Answer from the drawing. Dimensions are ordinates in mm from the lowest x, y and z of the part. Round coordinates to 2 decimals unless told otherwise and drop trailing zeros. Write each loop counter-clockwise with the first axis right and the second up, starting at its lowest first coordinate (ties: lowest second). Pieces come first, ordered by that corner, then holes. Notation, with made-up numbers: (22, 35.5) - (51, 35.5) arc R14 cw to (51, 55.5) - close; hole circle Ø1 at (56.5, 39.5). An arc over 180 degrees is marked (long way). Return JSON: item names as keys, results as strings. Group by question number.
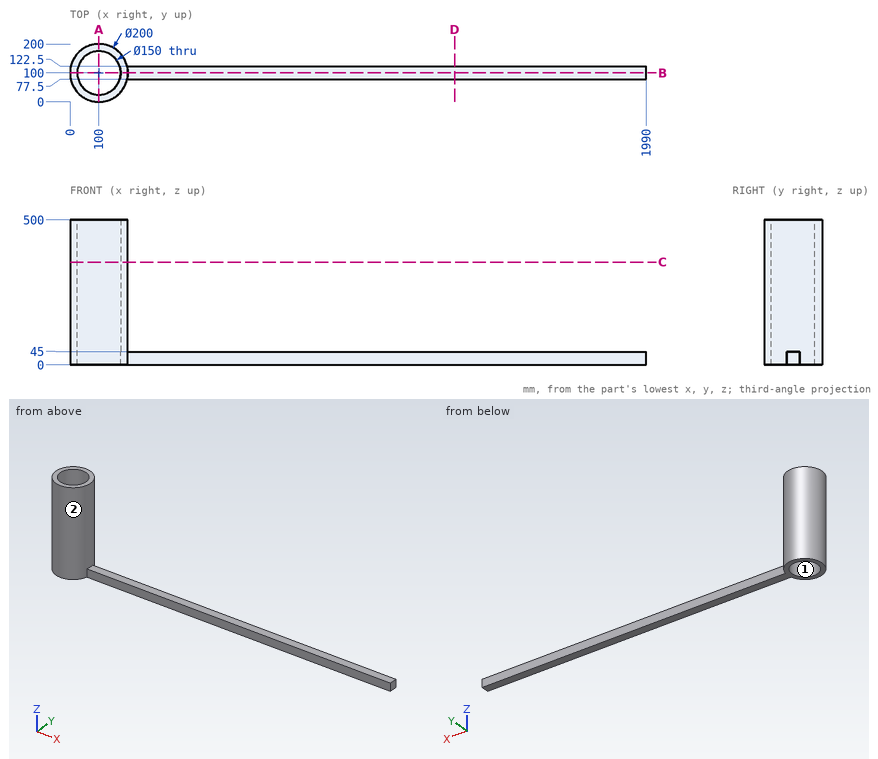
(1) Determine the mould class of the marked faces 1 and 2 for opening direction Y: +Y half, -Y half, draft (parallel to the pull), parting line (faces both ways), or undercut.
(2) Find section A-A (x = 100). Write down the section's boundary in (y, z), plus the area to 3 significant figures.
(3) Find section D-D (x = 1329). Write down the section's boundary in (y, z).
(4) Find section C-C (z = 354.5). Write down the section's boundary in (x, y).
(5) Find section B-B (y = 100). Write down the section's boundary in (x, z), plus the area to 3 significant figures.
(6) Flat-ended cylindrical pins translate along their axes: pin 1 (2 mm diameter, centred on y = 86, z = 366.5, fed in from +X); pin 2 (8 mm diameter, centred on y = 167.5, z = 224.5, fed in from +X); pin 3 (5 mm diameter, centred on y = 21, z = 77, fed in from -X). Find the tip coordinate at first contact, or state that the pin passes through.
(7) Consider line 1 (Y direction, x = 100, z = 325); line 2 (X direction, y = 95, z = 201.5); line 3 (Z direction, x = 355, y = 78.5). Determine where each line is inside the solid, lowest interval first.
Check sheet entries:
{
 "1": {"face 1": "undercut", "face 2": "parting line"},
 "2": {"outline": "(0, 0) - (25, 0) - (25, 500) - (0, 500) - close; (175, 0) - (200, 0) - (200, 500) - (175, 500) - close", "area": "25,000 mm^2"},
 "3": {"outline": "(77.5, 0) - (122.5, 0) - (122.5, 45) - (77.5, 45) - close"},
 "4": {"outline": "circle Ø200 at (100, 100); hole circle Ø150 at (100, 100)"},
 "5": {"outline": "(0, 0) - (25, 0) - (25, 500) - (0, 500) - close; (175, 0) - (1990, 0) - (1990, 45) - (200, 45) - (200, 500) - (175, 500) - close", "area": "106,000 mm^2"},
 "6": {"pin 1": "stops at x = 199.15", "pin 2": "stops at x = 177.25", "pin 3": "stops at x = 35.6"},
 "7": {"line 1": "y = 0 to 25, 175 to 200", "line 2": "x = 0.13 to 25.17, 174.83 to 199.87", "line 3": "z = 0 to 45"}
}
